Design review of the part built by this model. Coordinates are the model's own, in mm. Round coordinates to 2 decimals unless told otherwise and drop trailing zeros. Order: outer loops, then holes, each group sorted by start corner. A loop starts at its lowest first (then second) coordinate and runs counter-clockwise, first axis right, second up. Notation, with made-up numbers: M -25,6.5 L 20,6.5 A24 ccw 20,35.5 Z; hole C 29.5,-22.5 d5. An arc over 180 degrees is marked long. Write item = value, one per line. Start each with the question number.
```python
from build123d import *

# Parameters (mm, degrees)
F0_W     = 2240.006
F0_H     = 732.282
F0_W_2   = 2080.006
F0_H_2   = 579.882
F1_DEPTH = 12.7
F2_D     = 4.7625


with BuildPart() as f1:
    # F0 (on Top) → F1 (new body)
    with BuildSketch(Plane.XY):
        Rectangle(F0_W, F0_H)
        Rectangle(F0_W_2, F0_H_2, mode=Mode.SUBTRACT)
    extrude(amount=F1_DEPTH)

    # F2 (through all)
    with Locations(Plane(origin=(0, 0, 0), x_dir=(1, 0, 0), z_dir=(0, 0, -1))):
        with Locations((-936.003, -329.941), (-792.003, -329.941), (-648.003, -329.941), (-504.003, -329.941), (-360.003, -329.941), (-1080.003, -329.941), (-1080.003, -197.9626), (-1080.003, -65.9842), (-1080.003, 197.9726), (-1080.003, 329.941), (-936.003, 329.941), (-792.003, 329.941), (-1080.003, 65.9942), (-648.003, 329.941), (-504.003, 329.941), (-360.003, 329.941), (-216.003, 329.941), (-72.003, 329.941), (215.997, 329.941), (71.997, 329.941), (359.997, 329.941), (503.997, 329.941), (647.997, 329.941), (791.997, 329.941), (935.997, 329.941), (1080.003, 329.941), (1079.997, 197.9626), (1079.997, 65.9842), (1079.997, -65.9942), (1079.997, -197.9726), (1079.997, -329.941), (935.997, -329.941), (791.997, -329.941), (647.997, -329.941), (503.997, -329.941), (359.997, -329.941), (215.997, -329.941), (71.997, -329.941), (-72.003, -329.941), (-216.003, -329.941), (-72.003, -329.941)):
            Hole(F2_D / 2)


solid = f1.part
```
(1) Consider section A-A, the plane x = -33. Write out the cut boundary in (y, z).
(2) Insertion check: pin 1 (4 mm diameter, centred on x = 1080.003, y = -329.941, fed in from -Z); pin 2 (6 mm diameter, centred on x = -216.003, y = 329.941, fed in from +Z). Each pin has a flat end and moves straight along its axis. Give the tip position at first contact, or say it passes through.
(3) For line 1 along X through (y, z) = (-168.5, 7.25); line 2 along Y through (x, z) = (532.5, 1.25), list the stretches that pass through material, from the lowest coordinate up. Write a range as [from, to].
(4) Consider section C-C, the plane z = 10.5. State how many separate pieces and enclosed holes the cut face has, then the cut area to 3 significant figures.
(5) Consider section B-B, the plane y = -252. Write out the cut boundary in (x, z), then the cut area to 3 significant figures.
Completed:
q1.outline = M -366.14,0 L -289.94,0 L -289.94,12.7 L -366.14,12.7 Z; M 289.94,0 L 366.14,0 L 366.14,12.7 L 289.94,12.7 Z
q2.pin_1 = through
q2.pin_2 = 12.7
q3.line_1 = [-1120, -1040], [1040, 1120]
q3.line_2 = [-366.14, -289.94], [289.94, 366.14]
q4.separate_pieces = 1
q4.enclosed_holes = 41
q4.area = 433,000 mm2
q5.outline = M -1120,0 L -1040,0 L -1040,12.7 L -1120,12.7 Z; M 1040,0 L 1120,0 L 1120,12.7 L 1040,12.7 Z
q5.area = 2,030 mm2
